from build123d import *

# Parameters (mm, degrees)
SKETCH1_W               = 13
SKETCH1_H               = 13
SKETCH1_W_2             = 11
SKETCH1_H_2             = 11
BOSS_EXTRUDE1_DEPTH     = 300
CUT_EXTRUDE2_DEPTH      = 1
CUT_EXTRUDE2_DEPTH_BACK = 14
CUT_EXTRUDE3_DEPTH      = 1
CUT_EXTRUDE3_DEPTH_BACK = 14


with BuildPart() as part:
    # Sketch1 → Boss-Extrude1 (new body)
    with BuildSketch(Plane.XY):
        Rectangle(SKETCH1_W, SKETCH1_H)
        Rectangle(SKETCH1_W_2, SKETCH1_H_2, mode=Mode.SUBTRACT)
    extrude(amount=BOSS_EXTRUDE1_DEPTH)

    # Sketch2 → Cut-Extrude2 (cut, two sides)
    with BuildSketch(Plane(origin=(6.5, 0, 0), x_dir=(0, 0, -1), z_dir=(1, 0, 0))) as cut_extrude2_sk:
        Polygon((12.787088063, 535.263128477), (-292.494446501, 6.5), (-300, -6.5), (-605.281534564, -535.263128477), (-1662.807791518, 75.299940651), (-1044.739168891, 1145.826197605), align=None)
    extrude(amount=CUT_EXTRUDE2_DEPTH, mode=Mode.SUBTRACT)
    extrude(cut_extrude2_sk.sketch, amount=-CUT_EXTRUDE2_DEPTH_BACK, mode=Mode.SUBTRACT)

    # Sketch3 → Cut-Extrude3 (cut, two sides)
    with BuildSketch(Plane(origin=(6.5, 0, 0), x_dir=(0, 0, -1), z_dir=(1, 0, 0))) as cut_extrude3_sk:
        Polygon((305.281534564, -535.263128477), (0, -6.5), (-7.505553499, 6.5), (-312.787088063, 535.263128477), (744.739168891, 1145.826197605), (1362.807791518, 75.299940651), align=None)
    extrude(amount=CUT_EXTRUDE3_DEPTH, mode=Mode.SUBTRACT)
    extrude(cut_extrude3_sk.sketch, amount=-CUT_EXTRUDE3_DEPTH_BACK, mode=Mode.SUBTRACT)


solid = part.part
Geometry: final body of the model. Coordinates: model frame, mm. A direction names the side the tool comes from. Coordinates: 2 decimals unless noted, no trailing zeros. Loops run counter-clockwise (first coordinate to the right, second up) from the corner with the lowest first, then second, coordinate; pieces in that order, holes last. Notation, with made-up numbers: (46.5, 12.25) - (99.5, 12.25) arc R20 ccw to (99.5, 19.25) - close; hole circle Ø7 at (65.5, 67). An arc over 180 degrees is marked (long way). One line per question, with ' | ' between items. Start each with the question number.
(1) Cut plane C-C on y = 3. Output: boundary loops of the cut face in (x, z).
(2) Cut plane A-A on z = 109. Output: boundary loops of the cut face in (x, y).
(3) Draft query along Y for faces 1 (the flat face through (6.5, 0, 148)), 2 (the flat face through (-5.687, 0.091, 296.195)), 3 (the flat face through (0, -5.5, 148)). Return one class per face: +Y half, -Y half, draft (parallel to the pull), parting line (faces both ways), or undercut.
(4) Ray query, L1, parallel to X at y = 2.5, z = 105.5; L2, parallel to Z at x = -6, y = -3. Return the intervals inside material, ascending. Write a range as from..to.
(5) Cut plane B-B on x = 3.5. Output: boundary loops of the cut face in (y, z).
(6) Reachability of faces 4 (the flat face through (0, 6.5, 148)), 5 (the flat face through (0, 5.5, 148)) from +Z, -Z, +X, -X, +Y, -Y: full face, straight path, thin tool, end or side. Return the list, or none.
Here are the results:
1) outline: (-6.5, 5.48) - (-5.5, 5.48) - (-5.5, 294.52) - (-6.5, 294.52) - close; (5.5, 5.48) - (6.5, 5.48) - (6.5, 294.52) - (5.5, 294.52) - close
2) outline: (-6.5, -6.5) - (6.5, -6.5) - (6.5, 6.5) - (-6.5, 6.5) - close; hole (-5.5, -5.5) - (5.5, -5.5) - (5.5, 5.5) - (-5.5, 5.5) - close
3) face 1: draft | face 2: +Y half | face 3: undercut
4) L1: -6.5..-5.5, 5.5..6.5 | L2: 2.02..297.98
5) outline: (-6.5, 0) - (-5.5, 0.58) - (-5.5, 299.42) - (-6.5, 300) - close; (5.5, 6.93) - (6.5, 7.51) - (6.5, 292.49) - (5.5, 293.07) - close
6) face 4: +Z, -Z, +X, -X, +Y | face 5: +Z, -Z
